Source: CAD feature listing. Evaluate the final solid. Frame: model axes, mm. Face numbers are marked on the shaded views. Give positions to 0.01 mm unless a question says otherwise; leave off trailing zeros. Order: outer loops, then holes, each group sorted by start corner. A loop starts at its lowest first (then second) coordinate and runs counter-clockwise, first axis right, second up. Notation, with made-up numbers: M -15,53 L 41,53 A23 ccw 41,76 Z; hole C 15,48 d8. An arc over 180 degrees is marked long. Answer in a Markdown table with one row per item. Add a question column.
(1) Material intervals for line 1 along X through (y, z) = (2.75, 5); line 2 along Y through (x, z) = (8, 6); line 3 along Z through (x, y) = (12, 6.5), sorted ascending.
(2) Section query C-C, the plane y = 4. Return loops of the section in (x, z), plus the area to 3 significant figures.
(3) Section query B-B, the plane z = 2.75. Return loops of the section in (x, y), plus the area to 3 significant figures.
(4) Mould query, pull axis Y, two halves, no side actions, for the marked faces 1, 2, 3 and 4. Classes: pulls with the +Y half, pulls with the -Y half, needs draft (parallel to the pull), parting line crosses it, or undercut.
(5) Pin query (flat end, axial travel): P1, Ø2, axis at x = 4, z = 5, coming from the +Y side; P2, Ø3, axis at x = 12, z = 5, coming from the +Y side; P3, Ø2, axis at x = 11, z = 3.5, coming from the +Y side; P4, Ø5.5, axis at x = 8, y = 52, coming from the +Z side (3 decimals). Return the tip coordinate at first contact, or that it passes through.
(6) Section query A-A, the plane x = 8. Return loops of the section in (y, z), plus the area to 3 significant figures.
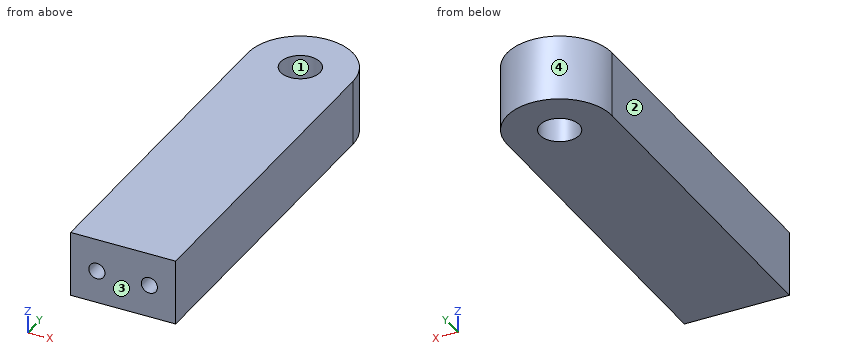
Autodesk Inventor part; units mm, degrees
ref_plane "YZ Plane" through (0, 0, 0) normal (1, 0, 0) x (0, 1, 0)
ref_plane "XZ Plane" through (0, 0, 0) normal (0, 1, 0) x (-1, 0, 0)
ref_plane "XY Plane" through (0, 0, 0) normal (0, 0, 1) x (1, 0, 0)
sketch "Sketch1" plane through (0, 0, 0) normal (0, 0, 1) x (1, 0, 0)
  line L0 (0, 0) -> (16, 0)
  line L1 (16, 0) -> (16, 60)
  line L2 (16, 60) -> (0, 60)
  line L3 (0, 60) -> (0, 0)
  circle A0 centre (8, 52) radius 3
  dimension "d9" = 16
  dimension "d10" = 60
  dimension "d11" = 6
  dimension "d12" = 8
extrude "Extrusion1" add sketch "Sketch1" along normal blind 10
sketch "Sketch2" plane through (0, 0, 10) normal (0, 0, 1) x (1, 0, 0)
  line L0 (16, 60) -> (0, 60)
  circle A0 centre (8, 52) radius 3
  arc A1 (16, 52) -> (0, 52) centre (8, 52) ccw
  line L1 (16.7201, 52) -> (16.7201, 60.3787)
  line L2 (16.7201, 60.3787) -> (-0.5009, 60.3787)
  line L3 (-0.5009, 60.3787) -> (-0.5009, 52)
  line L4 (-0.5009, 52) -> (0, 52)
  line L5 (16, 52) -> (16.7201, 52)
  point P0 (0, 0)
extrude "Extrusion2" cut sketch "Sketch2" against normal up to next contours A1 L4 L3 L2 L1 L5
sketch "Sketch3" plane through (0, 0, 0) normal (0, -1, 0) x (1, 0, 0)
  line L0 (0, 10) -> (16, 10)
  line L1 (0, 0) -> (16, 0)
  line L2 (0, 0) -> (0, 10)
  line L3 (16, 0) -> (16, 10)
  point P0 (4, 5)
  point P1 (12, 5)
  dimension "d19" = 5
  dimension "d20" = 5
  dimension "d21" = 4
  dimension "d22" = 4
hole "Hole1" at (4, 0, 5) at (12, 0, 5) direction (0, 1, 0) diameter 2.459 depth 8.8 tip angle 118
properties part number "SupportCylinder"
Values follow:
| question | item | result |
|---|---|---|
| 1 | line 1 | x = 0 to 2.77, 5.23 to 10.77, 13.23 to 16 |
| 1 | line 2 | y = 0 to 49, 55 to 60 |
| 1 | line 3 | z = 0 to 3.77, 6.23 to 10 |
| 2 | outline | M 0,0 L 16,0 L 16,10 L 0,10 Z; hole C 4,5 d2.46; hole C 12,5 d2.46 |
| 2 | area | 151 mm² |
| 3 | outline | M 0,0 L 16,0 L 16,52 A8 ccw 0,52 Z; hole C 8,52 d6 |
| 3 | area | 904 mm² |
| 4 | face 1 | undercut |
| 4 | face 2 | needs draft |
| 4 | face 3 | pulls with the -Y half |
| 4 | face 4 | pulls with the +Y half |
| 5 | P1 | stops at y = 59.42 |
| 5 | P2 | stops at y = 59.6 |
| 5 | P3 | stops at y = 59.75 |
| 5 | P4 | passes through |
| 6 | outline | M 0,0 L 49,0 L 49,10 L 0,10 Z; M 55,0 L 60,0 L 60,10 L 55,10 Z |
| 6 | area | 540 mm² |
